```python
from build123d import *

# Parameters (mm, degrees)
SKETCH2_W           = 15
SKETCH2_H           = 50
CUT_EXTRUDE1_DEPTH  = 1
SKETCH5_W           = 15
SKETCH5_H           = 8
BOSS_EXTRUDE1_DEPTH = 15


with BuildPart() as part:
    # Sketch1 → Revolve7 (revolve)
    with BuildSketch(Plane(origin=(0, 0, 0), x_dir=(0, 0, -1), z_dir=(1, 0, 0))):
        with BuildLine():
            Line((-61.371087, -39.717122139), (-27.130920736, 18.231080979))
            ThreePointArc((-27.130920736, 18.231080979), (-17.689796022, 29.084281592), (-5, 35.858931127))
            Line((-5, 35.858931127), (-5, 45))
            Line((-5, 45), (-8, 45))
            Line((-8, 45), (-8, 37.992245332))
            ThreePointArc((-8, 37.992245332), (-20.415266058, 30.730416935), (-29.713738459, 19.757204371))
            Line((-29.713738459, 19.757204371), (-60.832382285, -32.908120885))
            ThreePointArc((-60.832382285, -32.908120885), (-63.651810303, -34.372652199), (-66.205866039, -32.482989368))
            Line((-66.205866039, -32.482989368), (-96.206333671, 43.558703481))
            Line((-96.206333671, 43.558703481), (-96.251196427, 45))
            Line((-96.251196427, 45), (-99.251196427, 45))
            Line((-99.251196427, 45), (-99.251196427, 43.102019876))
            Line((-99.251196427, 43.102019876), (-66.744570754, -39.291990621))
            ThreePointArc((-66.744570754, -39.291990621), (-64.190515018, -41.181653452), (-61.371087, -39.717122139))
        make_face()
    revolve(axis=Axis((0, 0, 0), (0, -1, 0)))

    # Sketch2 → Cut-Extrude1 (cut)
    with BuildSketch(Plane(origin=(0, 18.126463109, -30.677303315), x_dir=(-1, 0, 0), z_dir=(0, 0.5087077972413765, -0.8609392411929117))):
        with Locations((0, -25)):
            Rectangle(SKETCH2_W, SKETCH2_H)
    extrude(amount=-CUT_EXTRUDE1_DEPTH, mode=Mode.SUBTRACT)

    # Sketch5 → Boss-Extrude1 (add)
    with BuildSketch(Plane(origin=(0, 17.617755312, -29.816364073), x_dir=(-1, 0, 0), z_dir=(0, 0.5087077972413765, -0.8609392411929117))):
        with Locations((0, -4)):
            Rectangle(SKETCH5_W, SKETCH5_H)
    extrude(amount=BOSS_EXTRUDE1_DEPTH)


solid = part.part
```
Verification items for the finished model (mm, model axes). A direction names the side the tool comes from. Round coordinates to 2 decimals unless told otherwise and drop trailing zeros. Write each loop counter-clockwise with the first axis right and the second up, starting at its lowest first coordinate (ties: lowest second). Pieces come first, ordered by that corner, then holes. Notation, with made-up numbers: (61, 59.5) - (83, 59.5) arc R23 ccw to (83, 81.5) - close; hole circle Ø2 at (-11, -0.75). An arc over 180 degrees is marked (long way). Answer as a JSON object with one key per item and string values. Group by question number.
Q1. Section check C-C, the plane y = 30. Give the number of separate pieces and of enclosed holes in the cut face, plus the area to 3 significant figures.
Q2. Mould release check, pull along X, two halves, no side actions. Record for faces 4 (the cylindrical face through (-29.81, 44.04, 94.67)), 5 (the flat face through (5.2, 45, 0.1)), 6 (the cylindrical face through (7.81, 41.45, -1.73)): released by +X, released by -X, zero draft, split by the parting line, or undercut.
Q3. Section check A-A, the plane y = -12. Enter the section's corners in (x, z), plus the area to 3 significant figures.
Q4. Go/stop test with flat-tipped pins: pin 1 Ø16 at (y, z) = (20.5, -35) entering from +X; pin 2 Ø1 at (y, z) = (33.5, 61) entering from +X; pin 3 Ø4 at (y, z) = (-12, -42.5) entering from -X. Record where each tip stops, or that it passes through.
Q5. Tool access check on faces 1 (the conical face through (43.771, -26.136, -57.085)), 2 (the flat face through (0.1, -7.1, -44.42)), 3 (the flat face through (7.5, 18, -38)). Record the directions out of +Z, -Z, +X, -X, +Y, -Y that give a thin tool (end or side, any length) a straight path to the whole face; none if there is none.
Q6. Thickness scan on line 1 (X direction, y = 39, z = 0); line 2 (X direction, y = -16, z = 11); line 3 (Z direction, x = -3, y = 1). Record the ranges inside material, lowest first.
Q7. Section check B-B, the plane y = 14. Enter the section's corners in (x, z).
Found:
{
 "1": {"separate pieces": "2", "enclosed holes": "2", "area": "2,440 mm^2"},
 "2": {"face 4": "split by the parting line", "face 5": "zero draft", "face 6": "undercut"},
 "3": {"outline": "circle Ø155.02 at (0, 0); (-7.5, -47.89) - (-7.5, -47.32) - (7.5, -47.32) - (7.5, -47.89) arc R48.48 ccw (long way) to start; hole circle Ø148.57 at (0, 0); hole circle Ø89.99 at (0, 0)", "area": "2,550 mm^2"},
 "4": {"pin 1": "stops at x = 87.82", "pin 2": "stops at x = 73.92", "pin 3": "stops at x = -66.4"},
 "5": {"face 1": "-Y", "face 2": "none", "face 3": "+Y"},
 "6": {"line 1": "x = -97.63 to -94.41, -8 to -5, 5 to 8, 94.41 to 97.63", "line 2": "x = -75.13 to -71.87, -49.64 to -46.06, 46.06 to 49.64, 71.87 to 75.13", "line 3": "z = -82.59 to -79.36, -39.64 to -37.19, 37.19 to 40.69, 79.36 to 82.59"},
 "7": {"outline": "circle Ø175.54 at (0, 0); (-7.5, -39.42) - (7.5, -39.42) - (7.5, -32.26) arc R33.12 ccw (long way) to (-7.5, -32.26) - close; hole circle Ø169.09 at (0, 0); hole circle Ø59.26 at (0, 0)"}
}
